```python
from build123d import *

# Parameters (mm, degrees)
F1_DEPTH       = 6
F3_D           = 6
F3_CSINK_D     = 9
F3_CSINK_ANGLE = 90
F5_D           = 3
F5_CSINK_D     = 4.5
F5_CSINK_ANGLE = 90


with BuildPart() as f1:
    # F0 (on Front) → F1 (new body)
    with BuildSketch(Plane.XZ):
        with BuildLine():
            Line((0, 170), (0, 0))
            Line((0, 0), (270, 47.6082847913))
            Line((270, 47.6082847913), (270, 63.3243455574))
            ThreePointArc((270, 63.3243455574), (268.2139380484, 67.154567773), (264.1317591117, 68.2483843224))
            Line((264.1317591117, 68.2483843224), (233.0388431092, 62.7658643223))
            ThreePointArc((233.0388431092, 62.7658643223), (212.7658643223, 76.9611568908), (226.9611568908, 97.2341356777))
            Line((226.9611568908, 97.2341356777), (264.2155372437, 103.8030880835))
            ThreePointArc((264.2155372437, 103.8030880835), (268.3623111018, 106.1972290868), (270, 110.6967423546))
            Line((270, 110.6967423546), (270, 164))
            Line((270, 164), (255, 164))
            Line((255, 164), (255, 170))
            Line((255, 170), (240, 170))
            Line((240, 170), (240, 164))
            Line((240, 164), (225, 164))
            Line((225, 164), (225, 170))
            Line((225, 170), (210, 170))
            Line((210, 170), (210, 164))
            Line((210, 164), (195, 164))
            Line((195, 164), (195, 170))
            Line((195, 170), (180, 170))
            Line((180, 170), (180, 164))
            Line((180, 164), (165, 164))
            Line((165, 164), (165, 170))
            Line((165, 170), (150, 170))
            Line((150, 170), (150, 164))
            Line((150, 164), (135, 164))
            Line((135, 164), (135, 170))
            Line((135, 170), (120, 170))
            Line((120, 170), (120, 164))
            Line((120, 164), (105, 164))
            Line((105, 164), (105, 170))
            Line((105, 170), (90, 170))
            Line((90, 170), (90, 164))
            Line((90, 164), (75, 164))
            Line((75, 164), (75, 170))
            Line((75, 170), (60, 170))
            Line((60, 170), (60, 164))
            Line((60, 164), (45, 164))
            Line((45, 164), (45, 170))
            Line((45, 170), (30, 170))
            Line((30, 170), (30, 164))
            Line((30, 164), (15, 164))
            Line((15, 164), (15, 170))
            Line((15, 170), (0, 170))
        make_face()
    extrude(amount=F1_DEPTH)

    # F3 (through all)
    with Locations(Plane.XZ.offset(6)):
        with Locations((12, 146), (12, 89), (12, 32)):
            CounterSinkHole(F3_D / 2, F3_CSINK_D / 2, counter_sink_angle=F3_CSINK_ANGLE)

    # F5 (through all)
    with Locations(Plane.XZ.offset(6)):
        with Locations((35, 116), (147.5, 116), (260, 116)):
            CounterSinkHole(F5_D / 2, F5_CSINK_D / 2, counter_sink_angle=F5_CSINK_ANGLE)


solid = f1.part
```
For this review, take the finished solid that the model builds, in its own axes (mm). A direction names the side the tool comes from. Coordinates: 2 decimals unless noted, no trailing zeros. Order: outer loops, then holes, each group sorted by start corner. A loop starts at its lowest first (then second) coordinate and runs counter-clockwise, first axis right, second up. Notation, with made-up numbers: (42.5, 51) -> (57.5, 51) arc R27 ccw to (57.5, 70) -> close; hole circle Ø8 at (-30, 23). An arc over 180 degrees is marked (long way). Answer as CSV lines item,"result".
Q1. We need section B-B (x = 12). State the section outline as (y, z) points.
Model answer:
outline,"(-6, 2.12) -> (0, 2.12) -> (0, 29) -> (-4.5, 29) -> (-6, 27.5) -> close; (-6, 36.5) -> (-4.5, 35) -> (0, 35) -> (0, 86) -> (-4.5, 86) -> (-6, 84.5) -> close; (-6, 93.5) -> (-4.5, 92) -> (0, 92) -> (0, 143) -> (-4.5, 143) -> (-6, 141.5) -> close; (-6, 150.5) -> (-4.5, 149) -> (0, 149) -> (0, 170) -> (-6, 170) -> close"
Q2. We need section D-D (z = 80). State the section outline as (x, y) points.
Model answer:
outline,"(0, -6) -> (212.5, -6) -> (212.5, 0) -> (0, 0) -> close"
Q3. Draft analysis for pull direction X (two halves, no side actions). For faces 3 (the face through (173, -3, 164)), 4 (the face through (98, -3, 170)), 5 (the face through (255, -3, 167)), state which applies: released by +X, released by -X, zero draft, split by the parting line, or undercut.
Model answer:
face 3,"undercut"
face 4,"zero draft"
face 5,"released by +X"
Q4. For faces 1 (the face through (203, -3, 164)), 2 (the face through (0, -3, 86)), list the 3-axis set-ups (+Z, -Z, +X, -X, +Y, -Y) from which the entire face can be reached by the end or side of a thin tool; tool diameter is ignored.
Model answer:
face 1,"+Z, +Y, -Y"
face 2,"+Z, -Z, -X, +Y, -Y"
Q5. Clearance check with flat-ended pins moving along their axes: pin 1 Ø1.8 at (y, z) = (-3, 167.5) entering from +X; pin 2 Ø1 at (x, y) = (40, -1.5) entering from -Z; pin 3 Ø4 at (x, z) = (35, 116) entering from -Y. State where each tip first meets the part, or that it passes through.
Model answer:
pin 1,"stops at x = 255"
pin 2,"stops at z = 6.96"
pin 3,"stops at y = -5.75"
Q6. We need section A-A (z = 146). State the section outline as (x, y) points, plus the area to 3 significant figures.
Model answer:
outline,"(0, -6) -> (7.5, -6) -> (9, -4.5) -> (9, 0) -> (0, 0) -> close; (15, -4.5) -> (16.5, -6) -> (270, -6) -> (270, 0) -> (15, 0) -> close"
area,"1,580 mm2"
Q7. We need section C-C (x = 230). State the section outline as (y, z) points, plus the area to 3 significant figures.
Model answer:
outline,"(-6, 40.56) -> (0, 40.56) -> (0, 62.5) -> (-6, 62.5) -> close; (-6, 97.77) -> (0, 97.77) -> (0, 164) -> (-6, 164) -> close"
area,"529 mm2"
Q8. Wall thickness on line 1 along X through (y, z) = (-2.95, 116); line 2 along X through (y, z) = (-2, 146); line 3 along Z through (x, y) = (12, -2.25): over which ranges is each line inside the solid? List them lowest first. Write a range as [from, to].
Model answer:
line 1,"x = [0, 33.5], [36.5, 146], [149, 258.5], [261.5, 270]"
line 2,"x = [0, 9], [15, 270]"
line 3,"z = [2.12, 29], [35, 86], [92, 143], [149, 170]"
